Source: CAD feature listing. Evaluate the final solid. Frame: model axes, mm. A direction names the side the tool comes from. Give positions to 0.01 mm unless a question says otherwise; leave off trailing zeros. Write each loop counter-clockwise with the first axis right and the second up, starting at its lowest first coordinate (ties: lowest second). Pieces come first, ordered by that corner, then holes. Notation, with made-up numbers: M 2,-38 L 61,-38 A18 cw 61,-13 Z; hole C 54.5,55.25 d11. An arc over 180 degrees is marked long. Return JSON: item names as keys, results as strings.
```python
from build123d import *

# Parameters (mm, degrees)
SKETCH1_W           = 73
SKETCH1_H           = 26
BOSS_EXTRUDE1_DEPTH = 5


with BuildPart() as part:
    # Sketch1 → Boss-Extrude1 (new body)
    with BuildSketch(Plane.XY):
        Polygon((64.038630962, -4.683293815), (69.038630962, -4.683293815), (69.038630962, 10.316706185), (64.038630962, 10.316706185), (64.038630962, 27.816706185), (69.044687612, 27.816706185), (69.044687612, 42.816706185), (-70.955312388, 42.816706185), (-70.955312388, 27.816706185), (-65.955312388, 27.816706185), (-65.955312388, 10.316706185), (-70.955312388, 10.316706185), (-70.955312388, -4.683293815), (-65.955312388, -4.683293815), (-65.955312388, -22.183293815), (-70.955312388, -22.183293815), (-70.955312388, -37.183293815), (-55.955312388, -37.183293815), (-55.955312388, -32.183293815), (-40.955312388, -32.183293815), (-40.955312388, -37.183293815), (-30.955312388, -37.183293815), (-30.955312388, -32.183293815), (-20.955312388, -32.183293815), (-20.955312388, -37.183293815), (-10.955312388, -37.183293815), (-10.955312388, -32.183293815), (-0.955312388, -32.183293815), (9.044687612, -32.183293815), (9.044687612, -37.183293815), (19.044687612, -37.183293815), (19.044687612, -32.183293815), (29.044687612, -32.183293815), (29.044687612, -37.183293815), (39.038630962, -37.183293815), (39.038630962, -32.183293815), (39.044687612, -32.183293815), (54.038630962, -32.183293815), (54.038630962, -37.183293815), (69.038630962, -37.183293815), (69.038630962, -22.183293815), (64.038630962, -22.183293815), align=None)
        with Locations((-0.955312388, 14.816706185)):
            Rectangle(SKETCH1_W, SKETCH1_H, mode=Mode.SUBTRACT)
    extrude(amount=BOSS_EXTRUDE1_DEPTH)


solid = part.part
```
1) Contact query for flat-ended pins moving along their axis: pin 1 Ø2.5 at (y, z) = (15, 3.5) entering from -X; pin 2 Ø1.5 at (y, z) = (-36, 1.5) entering from +X; pin 3 Ø2.5 at (y, z) = (22.5, 3.5) entering from +X; pin 4 Ø3 at (x, y) = (-56, -10.5) entering from -Z. Output: stop coordinate, or through.
Numbers:
{"pin 1": "stops at x = -65.96", "pin 2": "stops at x = 69.04", "pin 3": "stops at x = 64.04", "pin 4": "stops at z = 0"}
2) Cut plane B-B, the plane x = -26. Return the cut outline in (y, z), then the cut area to 3 significant figures.
Numbers:
{"outline": "M -32.18,0 L 1.82,0 L 1.82,5 L -32.18,5 Z; M 27.82,0 L 42.82,0 L 42.82,5 L 27.82,5 Z", "area": "245 mm²"}
3) Set-up query: faces 1 (the face through (-1, 27.817, 2)), 2 (the face through (-26, -32.183, 2)), 3 (the face through (-65.955, -13, 2)), 4 (the face through (67, 10.317, 2)). Return all of +Z, -Z, +X, -X, +Y, -Y with unobstructed straight access to the full face (end or side cutting, diameter ignored); none if empty.
Numbers:
{"face 1": "+Z, -Z", "face 2": "+Z, -Z, -Y", "face 3": "+Z, -Z, -X", "face 4": "+Z, -Z, +X"}
4) Line query: line 1 (Y direction, x = -22, z = 1.85); line 2 (Y direction, x = 9.5, z = 3.4); line 3 (X direction, y = 12.5, z = 3.15). Output: solid intervals per line, ascending. Write a range as [from, to].
Numbers:
{"line 1": "y = [-32.18, 1.82], [27.82, 42.82]", "line 2": "y = [-37.18, 1.82], [27.82, 42.82]", "line 3": "x = [-65.96, -37.46], [35.54, 64.04]"}
5) Cut plane A-A, the plane y = 17.5. Return the cut outline in (x, z), then the cut area to 3 significant figures.
Numbers:
{"outline": "M -65.96,0 L -37.46,0 L -37.46,5 L -65.96,5 Z; M 35.54,0 L 64.04,0 L 64.04,5 L 35.54,5 Z", "area": "285 mm²"}
6) Cut plane D-D, the plane y = -19. Return the cut outline in (x, z), then the cut area to 3 significant figures.
Numbers:
{"outline": "M -65.96,0 L 64.04,0 L 64.04,5 L -65.96,5 Z", "area": "650 mm²"}
7) Cut plane C-C, the plane x = 46. Return the cut outline in (y, z), then the cut area to 3 significant figures.
Numbers:
{"outline": "M -32.18,0 L 42.82,0 L 42.82,5 L -32.18,5 Z", "area": "375 mm²"}
